The listing builds one solid part. Answer for the finished solid, in the listing's coordinates (mm). Give positions to 0.01 mm unless a question says otherwise; leave off trailing zeros. Write each loop counter-clockwise with the first axis right and the second up, starting at its lowest first coordinate (ties: lowest second). Pieces come first, ordered by that corner, then holes. Notation, with made-up numbers: (2, 10.5) - (40, 10.5) arc R17 ccw to (40, 28.5) - close; hole circle Ø2 at (-36, 51). An arc over 180 degrees is marked (long way). Return JSON: item names as keys, results as strings.
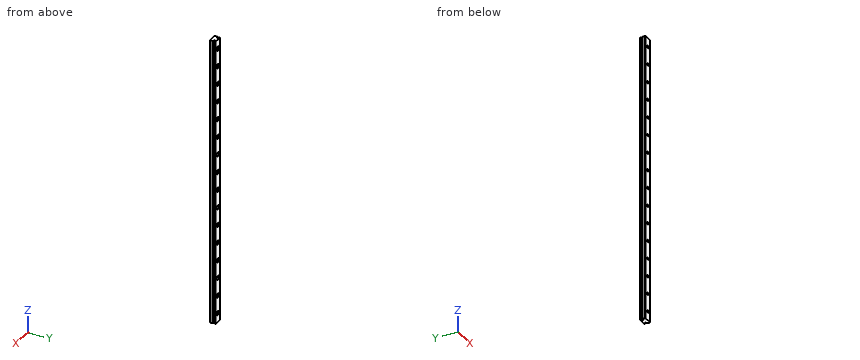
from build123d import *

# Parameters (mm, degrees)
EXTRUDE_1_DEPTH           = 400
HOLE_WIZARD_4_D           = 3.5
HOLE_WIZARD_4_CBORE_D     = 5.8
HOLE_WIZARD_4_CBORE_DEPTH = 4.5
HOLE_WIZARD_3_D           = 3.5
HOLE_WIZARD_3_DEPTH       = 7.916912277
HOLE_WIZARD_3_CBORE_D     = 5.8
HOLE_WIZARD_3_CBORE_DEPTH = 4.5


with BuildPart() as part:
    # 草图1 → 凸台-拉伸1 (new body)
    with BuildSketch(Plane.XY):
        Polygon((5.617628384, 4.221881307), (16.617628384, 4.221881307), (17.117628384, 4.721881307), (17.117628384, 8.221881307), (14.117628384, 9.445409037), (14.117628384, 9.987809251), (17.117628384, 11.343384147), (17.117628384, 11.721881307), (16.617628384, 12.221881307), (5.617628384, 12.221881307), (5.117628384, 11.721881307), (5.117628384, 11.211336981), (8.117628384, 9.987809251), (8.117628384, 9.445409037), (5.117628384, 8.221881307), (5.117628384, 4.721881307), align=None)
    extrude(amount=EXTRUDE_1_DEPTH)

    # 孔4 (through all)
    with Locations(Plane(origin=(11.117628384, 12.221881307, 387.5), x_dir=(0, 0, 1), z_dir=(0, 1, 0))):
        with Locations((0, 0), (-25, 0), (-49.975489716, 0), (-75, 0), (-100, 0), (-125.000497417, 0), (-150, 0), (-175, 0), (-200, 0), (-225, 0), (-250, 0), (-275, 0), (-300, 0), (-325, 0), (-350, 0), (-375, 0)):
            CounterBoreHole(HOLE_WIZARD_4_D / 2, HOLE_WIZARD_4_CBORE_D / 2, HOLE_WIZARD_4_CBORE_DEPTH)

    # 孔3
    with Locations(Plane(origin=(11.117628384, 12.221881307, 387.223861755), x_dir=(0, 0, 1), z_dir=(0, 1, 0))):
        with Locations((0, 0)):
            CounterBoreHole(HOLE_WIZARD_3_D / 2, HOLE_WIZARD_3_CBORE_D / 2, HOLE_WIZARD_3_CBORE_DEPTH, depth=HOLE_WIZARD_3_DEPTH)


solid = part.part
Item 1: Consider L1, parallel to X at y = 5.5, z = 336; L2, parallel to Y at x = 16.75, z = 218; L3, parallel to X at y = 10, z = 286. Determine where each line is inside the solid, lowest interval first.
Answer below:
{"L1": "x = 5.12 to 10.26, 11.98 to 17.12", "L2": "y = 4.35 to 8.37, 11.18 to 12.09", "L3": "x = 8.09 to 8.64, 13.6 to 14.14"}
Item 2: Flat-ended cylindrical pins translate along their axes: P1, Ø5, axis at x = 11.12, z = 112.5, coming from the +Y side; P2, Ø6.5, axis at x = 11.12, z = 337.52, coming from the -Y side. Find the tip coordinate at first contact, or state that the pin passes through.
Answer below:
{"P1": "stops at y = 7.72", "P2": "stops at y = 4.22"}
Item 3: A cutting plane is placed at A-A on z = 271. Determine the outline of the cut face in (x, y), then the cut area to 3 significant figures.
Answer below:
{"outline": "(5.12, 4.72) - (5.62, 4.22) - (16.62, 4.22) - (17.12, 4.72) - (17.12, 8.22) - (14.12, 9.45) - (14.12, 9.99) - (17.12, 11.34) - (17.12, 11.72) - (16.62, 12.22) - (5.62, 12.22) - (5.12, 11.72) - (5.12, 11.21) - (8.12, 9.99) - (8.12, 9.45) - (5.12, 8.22) - close", "area": "84.7 mm²"}
